from build123d import *

# Parameters (mm, degrees)
SKETCH1_W                = 76.2
SKETCH1_H                = 25.4
BOSS_EXTRUDE1_DEPTH      = 6.35
BOSS_EXTRUDE1_DEPTH_BACK = 6.35
SKETCH4_W                = 6.35
SKETCH4_H                = 25.4
BOSS_EXTRUDE3_DEPTH      = 6.35
SKETCH6_R                = 1.5113
CUT_EXTRUDE1_DEPTH       = 13.7


with BuildPart() as part:
    # Sketch1 → Boss-Extrude1 (new body, two sides)
    with BuildSketch(Plane.XY) as boss_extrude1_sk:
        Rectangle(SKETCH1_W, SKETCH1_H)
    extrude(amount=BOSS_EXTRUDE1_DEPTH)
    extrude(boss_extrude1_sk.sketch, amount=-BOSS_EXTRUDE1_DEPTH_BACK)

    # Sketch4 → Boss-Extrude3 (add)
    with BuildSketch(Plane.XY.offset(6.35)):
        with Locations((-28.575, 0)):
            Rectangle(SKETCH4_W, SKETCH4_H)
        with Locations((28.575, 0)):
            Rectangle(SKETCH4_W, SKETCH4_H)
    extrude(amount=BOSS_EXTRUDE3_DEPTH)

    # Sketch6 → Cut-Extrude1 (cut, through all)
    with BuildSketch(Plane.XY.offset(6.35)):
        Circle(SKETCH6_R)
    extrude(amount=-CUT_EXTRUDE1_DEPTH, mode=Mode.SUBTRACT)


solid = part.part
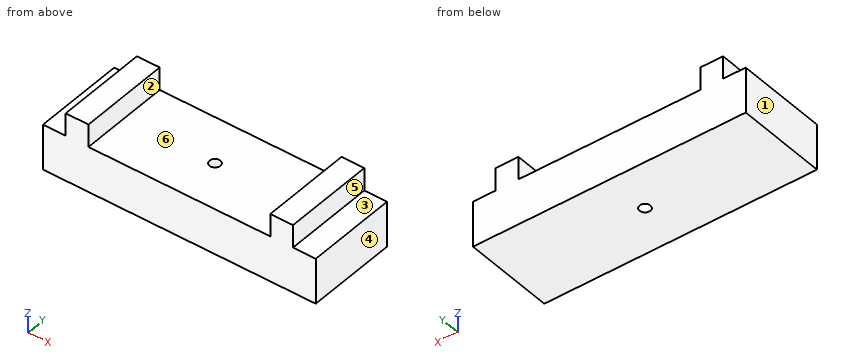
For this review, take the finished solid that the model builds, in its own axes (mm). Face numbers are marked on the shaded views. A direction names the side the tool comes from. Give positions to 0.01 mm unless a question says otherwise; leave off trailing zeros. Loops run counter-clockwise (first coordinate to the right, second up) from the corner with the lowest first, then second, coordinate; pieces in that order, holes last. Notation, with made-up numbers: M 74.5,80.25 L 113.5,80.25 A19 ccw 113.5,105.25 Z; hole C 62.25,-13.75 d5. An arc over 180 degrees is marked long. Put each result on its own line as item: value. Start each with the question number.
(1) Add section A-A, the plane z = 8.25. Write out the cut boundary in (x, y), then the cut area to 3 significant figures.
(2) Add section B-B, the plane x = 0. Write out the cut boundary in (y, z), then the cut area to 3 significant figures.
(3) Add section D-D, the plane y = 11. Write out the cut boundary in (x, z).
(4) The part is to be moulded in two halves that separate along X. For the marked faces 1, 2 and 3, say which applies: +X half, -X half, draft (parallel to the pull), parting line (faces both ways), or undercut.
(5) For pin 1 (1.9 mm diameter, centred on y = 2.5, z = 9.5, fed in from +X); pin 2 (10 mm diameter, centred on x = 12.5, y = 0, fed in from +Z); pin 3 (1.9 mm diameter, centred on y = -5, z = 8.5, fed in from -X), all flat-tipped, find the tip position at first contact; note any pin that passes through.
(6) Add section C-C, the plane y = 0. Write out the cut boundary in (x, z).
(7) Wall thickness on L1, parallel to Y at x = 0, z = -2.25; L2, parallel to Z at x = -20.5, y = -10.25; L3, parallel to X at y = 9, z = 8.75: over which ranges is each line inside the solid? List them lowest first.
(8) Machinability: for the marked faces 4, 5 and 6, which of the approach directions +Z, -Z, +X, -X, +Y, -Y give a long, thin tool a straight path to every point of the face, cutting with its end or side? Answer none if there is none.
Result:
1. outline: M -31.75,-12.7 L -25.4,-12.7 L -25.4,12.7 L -31.75,12.7 Z; M 25.4,-12.7 L 31.75,-12.7 L 31.75,12.7 L 25.4,12.7 Z
1. area: 323 mm^2
2. outline: M -12.7,-6.35 L -1.51,-6.35 L -1.51,6.35 L -12.7,6.35 Z; M 1.51,-6.35 L 12.7,-6.35 L 12.7,6.35 L 1.51,6.35 Z
2. area: 284 mm^2
3. outline: M -38.1,-6.35 L 38.1,-6.35 L 38.1,6.35 L 31.75,6.35 L 31.75,12.7 L 25.4,12.7 L 25.4,6.35 L -25.4,6.35 L -25.4,12.7 L -31.75,12.7 L -31.75,6.35 L -38.1,6.35 Z
4. face 1: -X half
4. face 2: undercut
4. face 3: draft
5. pin 1: stops at x = 31.75
5. pin 2: stops at z = 6.35
5. pin 3: stops at x = -31.75
6. outline: M -38.1,-6.35 L -1.51,-6.35 L -1.51,6.35 L -25.4,6.35 L -25.4,12.7 L -31.75,12.7 L -31.75,6.35 L -38.1,6.35 Z; M 1.51,-6.35 L 38.1,-6.35 L 38.1,6.35 L 31.75,6.35 L 31.75,12.7 L 25.4,12.7 L 25.4,6.35 L 1.51,6.35 Z
7. L1: y = -12.7 to -1.51, 1.51 to 12.7
7. L2: z = -6.35 to 6.35
7. L3: x = -31.75 to -25.4, 25.4 to 31.75
8. face 4: +Z, -Z, +X, +Y, -Y
8. face 5: +Z, +X, +Y, -Y
8. face 6: +Z, +Y, -Y
